Source: CAD feature listing. Evaluate the final solid. Frame: model axes, mm. Face numbers are marked on the shaded views. Coordinates: 2 decimals unless noted, no trailing zeros. Write each loop counter-clockwise with the first axis right and the second up, starting at its lowest first coordinate (ties: lowest second). Pieces come first, ordered by that corner, then holes. Notation, with made-up numbers: (47, 41.5) - (88, 41.5) arc R22 cw to (88, 77.5) - close; hole circle Ø4 at (32, -17.75). An arc over 180 degrees is marked (long way). One line per question, with ' | ' between items.
from build123d import *

# Parameters (mm, degrees)
SKETCH1_R           = 6
SKETCH1_R_2         = 3
BOSS_EXTRUDE1_DEPTH = 9.5
SKETCH2_W           = 0.770034963
SKETCH2_H           = 1.2
CHAMFER1_SIZE       = 0.3


with BuildPart() as part:
    # Sketch1 → Boss-Extrude1 (new, symmetric)
    with BuildSketch(Plane(origin=(0, 0, 0), x_dir=(1, 0, 0), z_dir=(0, 1, 0))):
        with Locations(Location((0, 0, 0), (0, 0, 270))):
            Circle(SKETCH1_R)
        with Locations(Location((0, 0, 0), (0, 0, 270))):
            Circle(SKETCH1_R_2, mode=Mode.SUBTRACT)
    extrude(amount=BOSS_EXTRUDE1_DEPTH, both=True)

    # Sketch2 → Cut-Revolve1 (revolve, cut)
    with BuildSketch(Plane(origin=(0, 0, 0), x_dir=(0, 0, -1), z_dir=(1, 0, 0)), mode=Mode.PRIVATE) as cut_revolve1_sk:
        with Locations((5.614982518, 5.9)):
            Rectangle(SKETCH2_W, SKETCH2_H)
        with Locations((5.614982518, -5.9)):
            Rectangle(SKETCH2_W, SKETCH2_H)
    revolve(cut_revolve1_sk.sketch.rotate(Axis((0, 9.5, 0), (0, -1, 0)), 180), axis=Axis((0, 9.5, 0), (0, -1, 0)), mode=Mode.SUBTRACT)

    # Chamfer1
    chamfer1_edges = [part.edges().sort_by_distance(p)[0] for p in [
        (0, -9.5, -6),
        (0, 9.5, -6),
        (0, -9.5, -3),
        (0, 9.5, -3),
    ]]
    chamfer(chamfer1_edges, length=CHAMFER1_SIZE)


solid = part.part
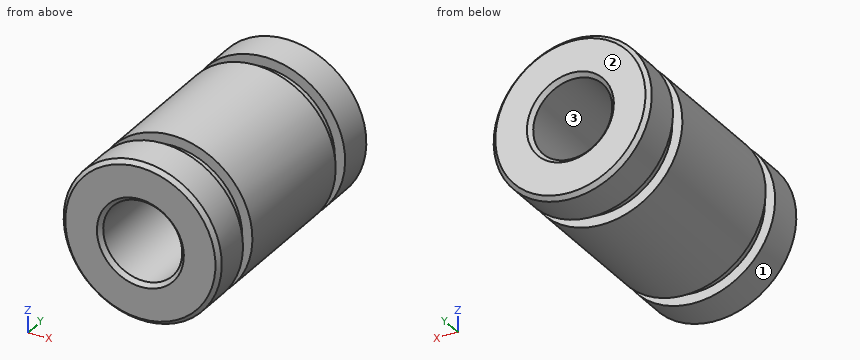
Item 1: Pin query (flat end, axial travel): pin 1 Ø1 at (x, z) = (-0.5, 2.5) entering from +Y; pin 2 Ø6 at (x, z) = (2, 0) entering from +Y; pin 3 Ø4 at (x, y) = (-3.5, 1) entering from +Z; pin 4 Ø2 at (y, z) = (-4.5, 3) entering from -X. Return the tip coordinate at first contact, or that it passes through.
Check sheet entries:
pin 1: y = 9.25 | pin 2: y = 9.5 | pin 3: z = 5.81 | pin 4: x = -5.66
Item 2: Cut plane C-C on y = -2.5. Return loops of the section in (x, z).
Check sheet entries:
outline: circle Ø12 at (0, 0); hole circle Ø6 at (0, 0)
Item 3: Mould query, pull axis Z, two halves, no side actions, for the marked faces 1, 2 and 3. Classes: pulls with the +Z half, pulls with the -Z half, needs draft (parallel to the pull), parting line crosses it, or undercut.
Check sheet entries:
face 1: parting line crosses it | face 2: needs draft | face 3: undercut
Item 4: Ray query, line 1 along Y through (x, z) = (-2.75, -4.5); line 2 along X through (y, z) = (-1, 0); line 3 along X through (y, z) = (5.75, 0). Return the intervals inside material, ascending. Write a range as [from, to].
Check sheet entries:
line 1: [-9.5, -6.5], [-5.3, 5.3], [6.5, 9.5] | line 2: [-6, -3], [3, 6] | line 3: [-5.23, -3], [3, 5.23]
